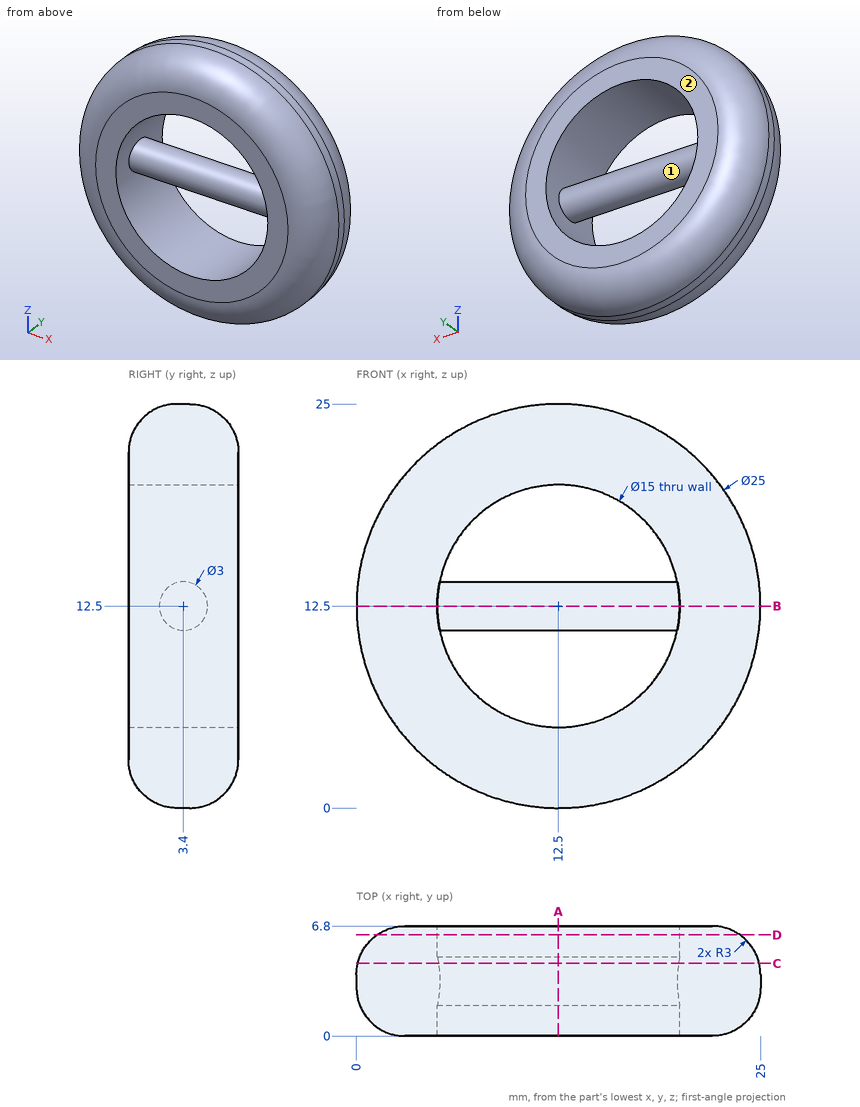
For this review, use the dimensioned drawing (mm, ordinates from the lowest corner) and the shaded views. A direction names the side the tool comes from. Give positions to 0.01 mm unless a question says otherwise; leave off trailing zeros. Order: outer loops, then holes, each group sorted by start corner. A loop starts at its lowest first (then second) coordinate and runs counter-clockwise, first axis right, second up. Notation, with made-up numbers: M 48.5,-38.5 L 74.5,-38.5 A24 cw 74.5,-25.5 Z; hole C -23,29.5 d10. An arc over 180 degrees is marked long. Use one line per item in the form item = value. Start each with the question number.
Item 1: Insertion check: pin 1 Ø1.5 at (x, y) = (13, 2) entering from +Z; pin 2 Ø3 at (x, y) = (21.5, 3) entering from +Z; pin 3 Ø3 at (y, z) = (1, 16) entering from +X. Each pin has a flat end and moves straight along its axis. Give the tip position at first contact, or say it passes through.
Item 2: To check wall thickness, follow line 1 along Z through (x, y) = (12.5, 3.25); line 2 along Z through (x, y) = (12.5, 2.5); line 3 along X through (y, z) = (3.75, 17). State the ranges of each line that lie inside material, in increasing order. Write a range as from..to.
Item 3: We need section B-B on z = 12.5. Give the boundary of the cut face in (x, y), plus the area to 3 significant figures.
Item 4: We need section A-A on x = 12.5. Give the boundary of the cut face in (y, z).
Item 5: We need section C-C on y = 4.5. Give the boundary of the cut face in (x, z).
Item 6: We need section D-D on y = 6.25. Give the boundary of the cut face in (x, z).
Item 7: For the marked faces 1 and 2, list the 3-axis set-ups (+Z, -Z, +X, -X, +Y, -Y) from which the entire face can be reached by the end or side of a thin tool; tool diameter is ignored.
Completed:
q1.pin_1 = 24.98
q1.pin_2 = 22.5
q1.pin_3 = 24.62
q2.line_1 = 0..5, 11.01..13.99, 20..25
q2.line_2 = 0.04..5, 11.3..13.7, 20..24.96
q2.line_3 = 0.84..6.5, 18.5..24.16
q3.outline = M 0,3 A3 ccw 3,0 L 5,0 L 5,1.9 L 20,1.9 L 20,0 L 22,0 A3 ccw 25,3 L 25,3.8 A3 ccw 22,6.8 L 20,6.8 L 20,4.9 L 5,4.9 L 5,6.8 L 3,6.8 A3 ccw 0,3.8 Z
q3.area = 105 mm²
q4.outline = M 0,3 A3 ccw 3,0 L 3.8,0 A3 ccw 6.8,3 L 6.8,5 L 0,5 Z; M 0,20 L 6.8,20 L 6.8,22 A3 ccw 3.8,25 L 3,25 A3 ccw 0,22 Z; C 3.4,12.5 d3
q5.outline = C 12.5,12.5 d24.83; hole M 5.07,11.48 A7.5 ccw 19.93,11.48 Z; hole M 5.07,13.52 L 19.93,13.52 A7.5 ccw Z
q6.outline = C 12.5,12.5 d22.46; hole C 12.5,12.5 d15
q7.face_1 = none
q7.face_2 = +Z, -Z, +X, -X, +Y
